Verification items for this drawing (mm, ordinates from the low corner). Give positions to 0.01 mm unless a question says otherwise; leave off trailing zeros. Loops run counter-clockwise (first coordinate to the right, second up) from the corner with the lowest first, then second, coordinate; pieces in that order, holes last. Notation, with made-up numbers: (25, 56.5) -> (59, 56.5) arc R27 ccw to (59, 78.5) -> close; hole circle Ø8 at (-26, 50). An arc over 180 degrees is marked (long way). Use one line per item in the form item = value. Start each with the question number.
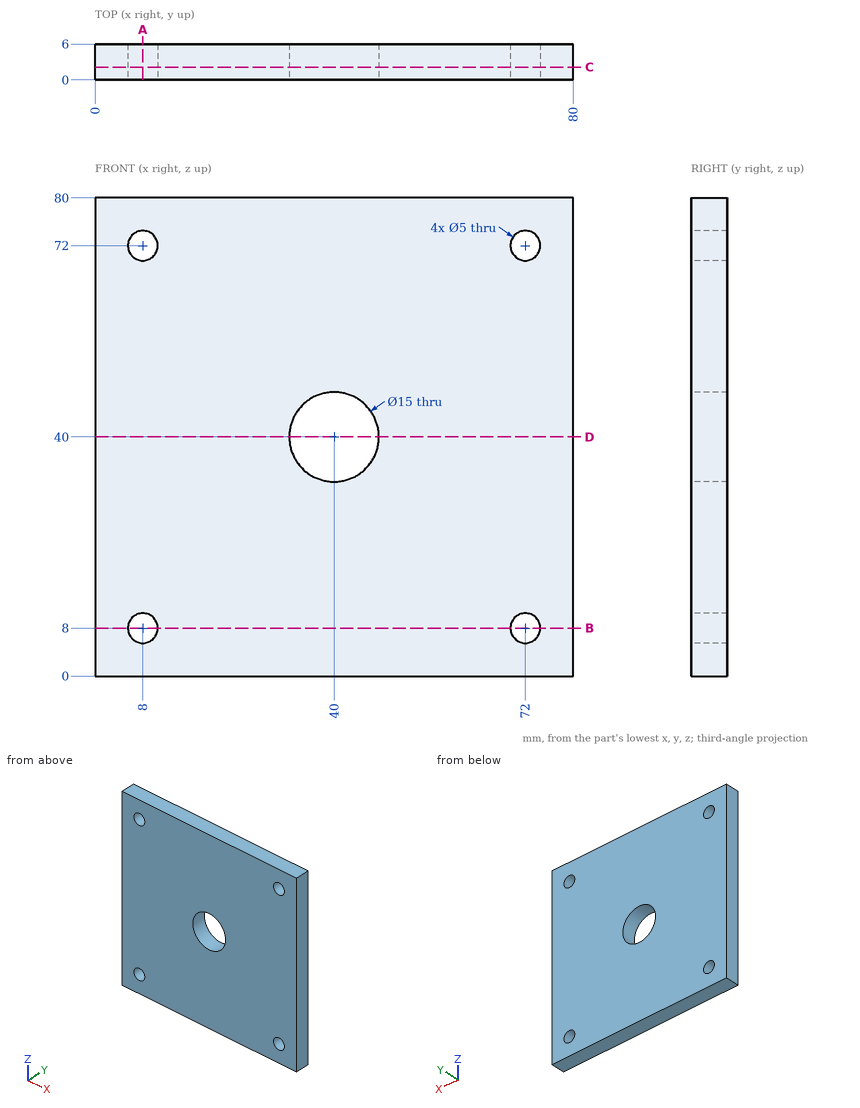
Item 1: Sectioned sample at D-D, the plane z = 40. Enter the section's corners in (x, y), and give its area (3 significant figures).
Item 2: Sectioned sample at B-B, the plane z = 8. Enter the section's corners in (x, y), and give its area (3 significant figures).
Item 3: Material ranges on line 1 (Z direction, x = 72, y = 3.1); line 2 (X direction, y = 4.6, z = 39.5), recorded low to high.
Item 4: Sectioned sample at C-C, the plane y = 2.15. Enter the section's corners in (x, z).
Item 5: Sectioned sample at A-A, the plane x = 8. Enter the section's corners in (y, z), and give its area (3 significant figures).
Outcome:
q1.outline = (0, 0) -> (32.5, 0) -> (32.5, 6) -> (0, 6) -> close; (47.5, 0) -> (80, 0) -> (80, 6) -> (47.5, 6) -> close
q1.area = 390 mm^2
q2.outline = (0, 0) -> (5.5, 0) -> (5.5, 6) -> (0, 6) -> close; (10.5, 0) -> (69.5, 0) -> (69.5, 6) -> (10.5, 6) -> close; (74.5, 0) -> (80, 0) -> (80, 6) -> (74.5, 6) -> close
q2.area = 420 mm^2
q3.line_1 = 0 to 5.5, 10.5 to 69.5, 74.5 to 80
q3.line_2 = 0 to 32.52, 47.48 to 80
q4.outline = (0, 0) -> (80, 0) -> (80, 80) -> (0, 80) -> close; hole circle Ø5 at (8, 8); hole circle Ø5 at (8, 72); hole circle Ø15 at (40, 40); hole circle Ø5 at (72, 8); hole circle Ø5 at (72, 72)
q5.outline = (0, 0) -> (6, 0) -> (6, 5.5) -> (0, 5.5) -> close; (0, 10.5) -> (6, 10.5) -> (6, 69.5) -> (0, 69.5) -> close; (0, 74.5) -> (6, 74.5) -> (6, 80) -> (0, 80) -> close
q5.area = 420 mm^2
